Geometry: final body of the model. Coordinates: model frame, mm. Round coordinates to 2 decimals unless told otherwise and drop trailing zeros. Loops run counter-clockwise (first coordinate to the right, second up) from the corner with the lowest first, then second, coordinate; pieces in that order, holes last. Notation, with made-up numbers: M 79,-8 L 88,-8 A20 ccw 88,26 Z; hole C 14,10 d7. An arc over 180 degrees is marked long. Return JSON: item names as keys, results as strings.
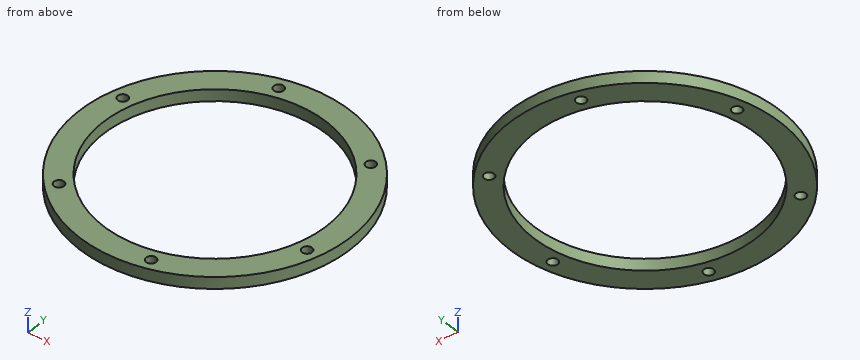
Solid Edge part; units mm, degrees
sketch "Sketch1" plane through (0, 0, 0) normal (0, 0, 1) x (1, 0, 0)
  circle A0 centre (0, 0) radius 38
  circle A1 centre (0, 0) radius 46.2
extrude "Protrusion1" add sketch "Sketch1" along normal blind 4
hole "Hole1" at (29.7692, 29.7692, 4) direction (0, 0, -1) diameter 3.4 end up to next
pattern_circular "Pattern1" count 6 over 360 about axis through (0, 0, 4) along (0, 0, -1) of "Hole1"
Q1. Section query C-C (x = 10.5). Output: boundary loops of the cut face in (y, z), plus the area to 3 significant figures.
Determined:
{"outline": "M -44.99,0 L -42.32,0 L -42.32,4 L -44.99,4 Z; M -39.01,0 L -36.52,0 L -36.52,4 L -39.01,4 Z; M 36.52,0 L 44.99,0 L 44.99,4 L 36.52,4 Z", "area": "54.5 mm^2"}
Q2. Section query D-D (z = 2.3). Output: boundary loops of the cut face in (x, y), plus the area to 3 significant figures.
Determined:
{"outline": "C 0,0 d92.4; hole C -40.67,10.9 d3.4; hole C 0,0 d76; hole C -29.77,-29.77 d3.4; hole C -10.9,40.67 d3.4; hole C 10.9,-40.67 d3.4; hole C 29.77,29.77 d3.4; hole C 40.67,-10.9 d3.4", "area": "2,110 mm^2"}
Q3. Section query A-A (x = 0). Output: boundary loops of the cut face in (y, z), plus the area to 3 significant figures.
Determined:
{"outline": "M -46.2,0 L -38,0 L -38,4 L -46.2,4 Z; M 38,0 L 46.2,0 L 46.2,4 L 38,4 Z", "area": "65.6 mm^2"}
Q4. Material intervals for L1, parallel to Y at x = 30, z = 0.2; L2, parallel to X at y = 1, z = 3.5; L3, parallel to Y at x = 0, z = 1.2, sorted ascending.
Determined:
{"L1": "y = -35.13 to -23.32, 23.32 to 28.08, 31.45 to 35.13", "L2": "x = -46.19 to -37.99, 37.99 to 46.19", "L3": "y = -46.2 to -38, 38 to 46.2"}
Q5. Pin query (flat end, axial travel): pin 1 (1 mm diameter, centred on y = 5.5, z = 1, fed in from +X). Return the tip coordinate at first contact, or that it passes through.
Determined:
{"pin 1": "stops at x = 45.93"}
